```python
from build123d import *

# Parameters (mm, degrees)
SKETCH1_R           = 6.35
BOSS_EXTRUDE1_DEPTH = 50.8
SKETCH6_R           = 4.7625
CUT_EXTRUDE3_DEPTH  = 12.7
SKETCH7_W           = 88.9
SKETCH7_H           = 38.1
CUT_EXTRUDE4_DEPTH  = 4.175
FILLET1_R           = 12.7
FILLET2_R           = 3.175


with BuildPart() as part:
    # Sketch1 → Boss-Extrude1 (new body)
    with BuildSketch(Plane.XY):
        with BuildLine():
            ThreePointArc((9.525, 0), (0, 9.525), (-9.525, 0))
            Line((-9.525, 0), (-9.525, -9.525))
            Line((-9.525, -9.525), (165.1, -9.525))
            Line((165.1, -9.525), (165.1, -6.35))
            Line((165.1, -6.35), (9.525, -6.35))
            Line((9.525, -6.35), (9.525, 0))
        make_face()
        Circle(SKETCH1_R, mode=Mode.SUBTRACT)
    boss_extrude1 = extrude(amount=BOSS_EXTRUDE1_DEPTH)

    # Sketch6 → Cut-Extrude3 (cut)
    with BuildSketch(Plane(origin=(0, -6.35, 0), x_dir=(1, 0, 0), z_dir=(0, 1, 0))):
        with Locations((22.225, -25.4)):
            Circle(SKETCH6_R)
        with Locations((101.6, -25.4)):
            Circle(SKETCH6_R)
    cut_extrude3 = extrude(amount=-CUT_EXTRUDE3_DEPTH, mode=Mode.SUBTRACT)

    # Mirror1: Boss-Extrude1, Cut-Extrude3 across plane
    add(boss_extrude1.mirror(Plane(origin=(165.1, 0, 50.8), x_dir=(0, 0, 1), z_dir=(1, 0, 0))))
    add(cut_extrude3.mirror(Plane(origin=(165.1, 0, 50.8), x_dir=(0, 0, 1), z_dir=(1, 0, 0))), mode=Mode.SUBTRACT)

    # Sketch7 → Cut-Extrude4 (cut, through all)
    with BuildSketch(Plane(origin=(0, -6.35, 0), x_dir=(1, 0, 0), z_dir=(0, 1, 0))):
        with Locations((165.1, -25.4)):
            Rectangle(SKETCH7_W, SKETCH7_H)
    extrude(amount=-CUT_EXTRUDE4_DEPTH, mode=Mode.SUBTRACT)

    # Fillet1
    fillet1_edges = [part.edges().sort_by_distance(p)[0] for p in [
        (120.65, -7.9375, 44.45),
        (120.65, -7.9375, 6.35),
        (209.55, -7.9375, 6.35),
        (209.55, -7.9375, 44.45),
    ]]
    fillet(fillet1_edges, radius=FILLET1_R)

    # Fillet2
    fillet2_edges = [part.edges().sort_by_distance(p)[0] for p in [
        (9.525, -6.35, 25.4),
        (320.675, -6.35, 25.4),
    ]]
    fillet(fillet2_edges, radius=FILLET2_R)


solid = part.part
```
Work out the finished part from the listing and answer in its coordinate system (mm). A direction names the side the tool comes from. Round coordinates to 2 decimals unless told otherwise and drop trailing zeros. Order: outer loops, then holes, each group sorted by start corner. A loop starts at its lowest first (then second) coordinate and runs counter-clockwise, first axis right, second up.
Q1. A cutting plane is placed at B-B, the plane z = 13. Determine the outline of the cut face in (x, y) (3 decimals).
Solution:
outline: (-9.525, -9.525) - (122.184, -9.525) - (122.184, -6.35) - (12.7, -6.35) arc R3.175 cw to (9.525, -3.175) - (9.525, 0) arc R9.525 ccw to (-9.525, 0) - close; (208.016, -9.525) - (339.725, -9.525) - (339.725, 0) arc R9.525 ccw to (320.675, 0) - (320.675, -3.175) arc R3.175 cw to (317.5, -6.35) - (208.016, -6.35) - close; hole circle Ø12.7 at (0, 0); hole circle Ø12.7 at (330.2, 0)
Q2. Find the intervals of material crossed by line 1 along Z through (x, y) = (228.6, -7.2); line 2 along X through (y, z) = (0.5, 11); line 3 along X through (y, z) = (-2.25, 10) (3 decimals), in increasing order.
Solution:
line 1: z = 0 to 20.64, 30.16 to 50.8
line 2: x = -9.51 to -6.33, 6.33 to 9.51, 320.69 to 323.87, 336.53 to 339.71
line 3: x = -9.525 to -5.938, 5.938 to 9.525, 320.675 to 324.262, 336.138 to 339.725
Q3. The mould has two halves that part along Z. Classify faces 3 (the flat face through (163, -6.35, 48)), 4 (the flat face through (179, -7, 0)), 5 (the cylindrical face through (100.98, -7.92, 20.68)), 6 (the cylindrical face through (224.057, -7.915, 23.969)): pulls with the +Z half, pulls with the -Z half, needs draft (parallel to the pull), parting line crosses it, or undercut.
Solution:
face 3: needs draft
face 4: pulls with the -Z half
face 5: undercut
face 6: undercut
Q4. Given pin 1 Ø4 at (y, z) = (3, 22) entering from +X; pin 2 Ø3 at (x, z) = (242.5, 8.5) entering from +Y; pin 3 Ø5 at (y, z) = (7, 21.5) entering from +X (3 decimals), each flat-ended and moving along its own axis, determine where each tip first touches the part or whether it passes through.
Solution:
pin 1: stops at x = 339.67
pin 2: stops at y = -6.35
pin 3: stops at x = 338.595
Q5. A cutting plane is placed at C-C, the plane x = 330.2. Determine the outline of the cut face in (y, z) (3 decimals), then the cut area to 3 significant figures.
Solution:
outline: (-9.525, 0) - (-6.35, 0) - (-6.35, 50.8) - (-9.525, 50.8) - close; (6.35, 0) - (9.525, 0) - (9.525, 50.8) - (6.35, 50.8) - close
area: 323 mm2
Q6. A tool of negligible diameter and unlimited length cuts with its end or side. For faces 1 (the flat face through (179, -7, 50.8)), 2 (the cylindrical face through (205.93, -7.96, 10.17)), from which of +Z, -Z, +X, -X, +Y, -Y can it reach the whole face along a straight path? Write none if from no direction.
Solution:
face 1: +Z, +X, -X, +Y, -Y
face 2: +Y, -Y
